```python
from build123d import *

# Parameters (mm, degrees)
SKETCH1_R           = 14
BOSS_EXTRUDE1_DEPTH = 1
SKETCH2_R           = 12.475
BOSS_EXTRUDE2_DEPTH = 7
SKETCH3_R           = 14
BOSS_EXTRUDE3_DEPTH = 1
SKETCH4_R           = 3.5
CUT_EXTRUDE1_DEPTH  = 22.748563171
SKETCH5_R           = 1.5
CUT_EXTRUDE2_DEPTH  = 22.748563171
CIRPATTERN1_COUNT   = 4


with BuildPart() as part:
    # Sketch1 → Boss-Extrude1 (new body)
    with BuildSketch(Plane(origin=(0, 0, 0), x_dir=(1, 0, 0), z_dir=(0, 1, 0))):
        with Locations(Location((0, 0, 0), (0, 0, 270))):
            Circle(SKETCH1_R)
    extrude(amount=BOSS_EXTRUDE1_DEPTH)

    # Sketch2 → Boss-Extrude2 (add)
    with BuildSketch(Plane(origin=(0, 1, 0), x_dir=(1, 0, 0), z_dir=(0, 1, 0))):
        with Locations(Location((0, 0, 0), (0, 0, 270))):
            Circle(SKETCH2_R)
    extrude(amount=BOSS_EXTRUDE2_DEPTH)

    # Sketch3 → Boss-Extrude3 (add)
    with BuildSketch(Plane(origin=(0, 8, 0), x_dir=(1, 0, 0), z_dir=(0, 1, 0))):
        with Locations(Location((0, 0, 0), (0, 0, 270))):
            Circle(SKETCH3_R)
    extrude(amount=BOSS_EXTRUDE3_DEPTH)

    # Sketch4 → Cut-Extrude1 (cut, through all)
    with BuildSketch(Plane(origin=(0, 9, 0), x_dir=(1, 0, 0), z_dir=(0, 1, 0))):
        with Locations(Location((0, 0, 0), (0, 0, 270))):
            Circle(SKETCH4_R)
    extrude(amount=-CUT_EXTRUDE1_DEPTH, mode=Mode.SUBTRACT)

    # Sketch5 → Cut-Extrude2 (cut, through all)
    with BuildSketch(Plane(origin=(0, 9, 0), x_dir=(1, 0, 0), z_dir=(0, 1, 0))):
        with Locations(Location((0, 9, 0), (0, 0, 270))):
            Circle(SKETCH5_R)
    cut_extrude2 = extrude(amount=-CUT_EXTRUDE2_DEPTH, mode=Mode.SUBTRACT)

    # CirPattern1: Cut-Extrude2 ×4 about axis
    cirpattern1_axis = Axis((0, 0, 0), (0, 1, 0))
    for i in range(1, CIRPATTERN1_COUNT):
        add(cut_extrude2.rotate(cirpattern1_axis, i * 360 / CIRPATTERN1_COUNT), mode=Mode.SUBTRACT)


solid = part.part
```
Geometry check sheet. Reference: the model listing, model coordinates, mm. A direction names the side the tool comes from. Give positions to 0.01 mm unless a question says otherwise; leave off trailing zeros. Loops run counter-clockwise (first coordinate to the right, second up) from the corner with the lowest first, then second, coordinate; pieces in that order, holes last. Notation, with made-up numbers: M -40,50 L -23,50 A22 ccw -23,87 Z; hole C -9.75,72.25 d9. An arc over 180 degrees is marked long. Write item = value, one per line. Start each with the question number.
1. Section check A-A, the plane x = 0. Enter the section's corners in (y, z) (3 decimals).
2. Section check B-B, the plane y = 8.5. Enter the section's corners in (x, z).
3. Thickness scan on probe 1 along X at (y, z) = (4.5, 1.25); probe 2 along X at (y, z) = (4.75, 2); probe 3 along Y at (x, z) = (12, -5.5). Record the ranges inside material, lowest first.
4. Section check C-C, the plane x = -9.5. Enter the section's corners in (y, z).
5. Draft check along Y on faces 3 (the face through (-0.07, 4.56, 10.5)), 4 (the face through (-3, 9, 3)), 5 (the face through (-1, 1, -13)). Enter one of: +Y half, -Y half, draft (parallel to the pull), parting line (faces both ways), or undercut.
6. Section check D-D, the plane z = 1. Enter the section's corners in (x, y), plus the area to 3 significant figures.
7. Go/stop test with flat-tipped pins: P1, Ø4, axis at y = 5, z = 10, coming from the +X side; P2, Ø5, axis at x = -9, z = 0, coming from the -Y side; P3, Ø1.8, axis at x = 9, z = 0, coming from the +Y side; P4, Ø1.5, axis at x = -10.5, y = 4.5, coming from the +Z side. Record where each tip stops, or that it passes through.
8. Tool access check on faces 1 (the face through (0.07, 4.56, -10.5)), 2 (the face through (10.519, 4.451, 6.706)). Record the directions out of +Z, -Z, +X, -X, +Y, -Y that give a thin tool (end or side, any length) a straight path to the whole face; none if there is none.
Values follow:
q1.outline = M 0,-14 L 1,-14 L 1,-12.475 L 8,-12.475 L 8,-14 L 9,-14 L 9,-10.5 L 0,-10.5 Z; M 0,-7.5 L 9,-7.5 L 9,-3.5 L 0,-3.5 Z; M 0,3.5 L 9,3.5 L 9,7.5 L 0,7.5 Z; M 0,10.5 L 9,10.5 L 9,14 L 8,14 L 8,12.475 L 1,12.475 L 1,14 L 0,14 Z
q2.outline = C 0,0 d28; hole C -9,0 d3; hole C 0,0 d7; hole C 0,-9 d3; hole C 0,9 d3; hole C 9,0 d3
q3.probe_1 = -12.41 to -9.83, -8.17 to -3.27, 3.27 to 8.17, 9.83 to 12.41
q3.probe_2 = -12.31 to -2.87, 2.87 to 12.31
q3.probe_3 = 0 to 1, 8 to 9
q4.outline = M 0,-10.28 L 1,-10.28 L 1,-8.09 L 8,-8.09 L 8,-10.28 L 9,-10.28 L 9,-1.41 L 0,-1.41 Z; M 0,1.41 L 9,1.41 L 9,10.28 L 8,10.28 L 8,8.09 L 1,8.09 L 1,10.28 L 0,10.28 Z
q5.face_3 = draft
q5.face_4 = +Y half
q5.face_5 = undercut
q6.outline = M -13.96,0 L -10.12,0 L -10.12,9 L -13.96,9 L -13.96,8 L -12.43,8 L -12.43,1 L -13.96,1 Z; M -7.88,0 L -3.35,0 L -3.35,9 L -7.88,9 Z; M 3.35,0 L 7.88,0 L 7.88,9 L 3.35,9 Z; M 10.12,0 L 13.96,0 L 13.96,1 L 12.43,1 L 12.43,8 L 13.96,8 L 13.96,9 L 10.12,9 Z
q6.area = 129 mm^2
q7.P1 = 9.57
q7.P2 = 0
q7.P3 = through
q7.P4 = 7.78
q8.face_1 = +Y, -Y
q8.face_2 = none
